Verification items for the finished model (mm, model axes). Face numbers are marked on the shaded views. A direction names the side the tool comes from. Coordinates: 2 decimals unless noted, no trailing zeros. Order: outer loops, then holes, each group sorted by start corner. A loop starts at its lowest first (then second) coordinate and runs counter-clockwise, first axis right, second up. Notation, with made-up numbers: (-1.5, -18.75) -> (30.5, -18.75) arc R8 ccw to (30.5, -3.75) -> close; hole circle Ø10 at (-1, 22.5). An arc over 180 degrees is marked (long way). Write item = value, one per line. Start each with the question number.
1. Cross-section at A-A on x = 0. Record the cut outline in (y, z), plus the area to 3 significant figures.
2. Thickness scan on line 1 along Y through (x, z) = (0, 3.75); line 2 along Z through (x, y) = (5, -4.75); line 3 along X through (y, z) = (0, 5.75). Record the ranges inside material, lowest first. Write a range as from..to.
3. Release check for a two-part mould opening along Y. For the marked faces 1, 2 and 3 record: +Y half, -Y half, draft (parallel to the pull), parting line (faces both ways), or undercut.
4. Cross-section at D-D on x = 3.5. Record the cut outline in (y, z).
5. Cross-section at C-C on y = -3.25. Record the cut outline in (x, z), plus the area to 3 significant figures.
6. Cross-section at B-B on x = 2.5. Record the cut outline in (y, z), plus the area to 4 significant figures.
7. Set-up check for the marked faces 4 and 5: record each of +Z, -Z, +X, -X, +Y, -Y from which the full face is reachable in a straight line by a thin tool's end or side.
8. Go/stop test with flat-tipped pins: P1, Ø2, axis at x = 1.5, z = 9.5, coming from the +Y side; P2, Ø5, axis at x = 5, z = 2, coming from the +Y side; P3, Ø3, axis at x = 4, z = 8, coming from the -Y side. Record where each tip stops, or that it passes through.
from build123d import *

# Parameters (mm, degrees)
BOSS_EXTRUDE2_DEPTH = 16
FILLET3_R           = 1
FILLET6_R           = 2
SKETCH7_W           = 5
SKETCH7_H           = 3
BOSS_EXTRUDE6_DEPTH = 1


with BuildPart() as part:
    # Sketch5 → Boss-Extrude2 (new body)
    with BuildSketch(Plane(origin=(4.228476288, 0, 0), x_dir=(1, 0, 0), z_dir=(0, 0, 1))):
        with BuildLine():
            Line((2.760085796, 0.4), (-3.422250513, 0.4))
            ThreePointArc((-3.422250513, 0.4), (-5.121328449, 0.113203437), (-3.547587232, -0.588549143))
            Line((-3.547587232, -0.588549143), (1.85826255, -3.462890458))
            Line((1.85826255, -3.462890458), (1.553106034, -4.036806393))
            Line((1.553106034, -4.036806393), (-3.378850655, -1.414438505))
            ThreePointArc((-3.378850655, -1.414438505), (-5.854676969, 0.279233492), (-2.955684082, 1.05))
            Line((-2.955684082, 1.05), (2.760085796, 1.05))
            Line((2.760085796, 1.05), (2.760085796, 0.4))
        make_face()
    extrude(amount=BOSS_EXTRUDE2_DEPTH)

    # Fillet3
    fillet3_edges = [part.edges().sort_by_distance(p)[0] for p in [
        (0.849625632, -1.414438505, 8),
        (1.272792206, 1.05, 8),
    ]]
    fillet(fillet3_edges, radius=FILLET3_R)

    # Fillet6
    fillet6_edges = [part.edges().sort_by_distance(p)[0] for p in [
        (0.680889056, -0.588549143, 8),
        (0.806225775, 0.4, 8),
    ]]
    fillet(fillet6_edges, radius=FILLET6_R)

    # Sketch7 → Boss-Extrude6 (add)
    with BuildSketch(Plane.XY.offset(16)):
        with Locations((4.488562084, 2.55)):
            Rectangle(SKETCH7_W, SKETCH7_H)
        Polygon((5.781582322, -4.036806393), (4.373167633, -6.685649172), (1.724324855, -5.277234484), (3.132739543, -2.628391705), align=None)
    extrude(amount=-BOSS_EXTRUDE6_DEPTH)


solid = part.part
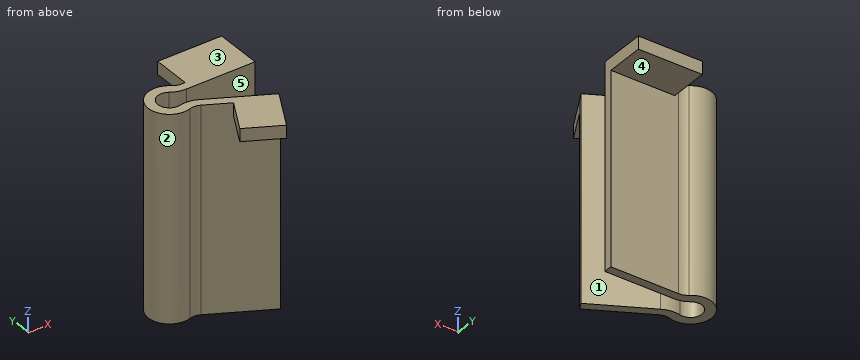
Worked out:
q1.outline = (-1.65, 0) -> (-0.9, 0) -> (-0.9, 16) -> (-1.65, 16) -> close; (0.9, 0) -> (1.65, 0) -> (1.65, 16) -> (0.9, 16) -> close
q1.area = 24.0 mm²
q2.line_1 = -1.65..-0.9, 0.9..1.65
q2.line_2 = 15..16
q2.line_3 = -1.65..-0.9
q3.face_1 = undercut
q3.face_2 = parting line
q3.face_3 = draft
q4.outline = (-6.22, 15) -> (-2.82, 15) -> (-2.82, 0) -> (-2.09, 0) -> (-2.09, 16) -> (-6.22, 16) -> close; (0.4, 0) -> (1.05, 0) -> (1.05, 15) -> (4.05, 15) -> (4.05, 16) -> (0.4, 16) -> close
q5.outline = (2.8, 15) -> (4.3, 15) -> (4.3, 0) -> (5.69, 0) -> (5.69, 16) -> (2.8, 16) -> close
q5.area = 23.7 mm²
q6.outline = (-5.69, 15) -> (-3.82, 15) -> (-3.82, 16) -> (-5.69, 16) -> close; (-2.29, 0) -> (-1.56, 0) -> (-1.56, 16) -> (-2.29, 16) -> close; (0.4, 0) -> (1.05, 0) -> (1.05, 15) -> (4.05, 15) -> (4.05, 16) -> (0.4, 16) -> close
q6.area = 27.05 mm²
q7.face_4 = -Z, +X, +Y
q7.face_5 = +Z, -Z, +X
q8.P1 = 1.57
q8.P2 = 1.05
q8.P3 = -3.89
